from build123d import *

# Parameters (mm, degrees)
SKETCH1_W           = 152.4
SKETCH1_H           = 76.2
BOSS_EXTRUDE1_DEPTH = 6.35
SKETCH2_W           = 6.35
SKETCH2_H           = 38.1
BOSS_EXTRUDE2_DEPTH = 6.35
CUT_EXTRUDE1_DEPTH  = 7.35
CUT_EXTRUDE2_DEPTH  = 7.35
BOSS_EXTRUDE3_DEPTH = 6.35
CUT_EXTRUDE3_DEPTH  = 7.35
FILLET1_R           = 48.26
CUT_EXTRUDE4_DEPTH  = 7.35
EXTRUDE_THIN2_DEPTH = 6.35
FILLET2_R           = 3.175


with BuildPart() as part:
    # Sketch1 → Boss-Extrude1 (new body)
    with BuildSketch(Plane.XY):
        with Locations((-76.2, -38.1)):
            Rectangle(SKETCH1_W, SKETCH1_H)
    extrude(amount=BOSS_EXTRUDE1_DEPTH)

    # Sketch2 → Boss-Extrude2 (add)
    with BuildSketch(Plane.XY.offset(6.35)):
        with Locations((3.175, -38.1)):
            Rectangle(SKETCH2_W, SKETCH2_H)
    extrude(amount=-BOSS_EXTRUDE2_DEPTH)

    # Sketch3 → Cut-Extrude1 (cut, through all)
    with BuildSketch(Plane.XY.offset(6.35)):
        Polygon((-152.4, -59.878913996), (-70.683723912, -12.7), (-12.7, -12.7), (-12.7, 0), (-152.4, 0), align=None)
    extrude(amount=-CUT_EXTRUDE1_DEPTH, mode=Mode.SUBTRACT)

    # Sketch4 → Cut-Extrude2 (cut, through all)
    with BuildSketch(Plane.XY.offset(6.35)):
        Polygon((-152.4, -59.878913996), (-133.35, -76.2), (-152.4, -76.2), align=None)
    extrude(amount=-CUT_EXTRUDE2_DEPTH, mode=Mode.SUBTRACT)

    # Sketch5 → Boss-Extrude3 (add)
    with BuildSketch(Plane.XY.offset(6.35)):
        Polygon((-87.181507854, -22.225), (-90.356507854, -16.725738686), (-123.352075739, -35.775738686), (-120.177075739, -41.275), align=None)
    extrude(amount=-BOSS_EXTRUDE3_DEPTH)

    # Sketch6 → Cut-Extrude3 (cut, through all)
    with BuildSketch(Plane.XY.offset(6.35)):
        Polygon((-134.802363795, -49.718913996), (-119.513501663, -76.2), (-133.35, -76.2), (-152.4, -59.878913996), align=None)
    extrude(amount=-CUT_EXTRUDE3_DEPTH, mode=Mode.SUBTRACT)

    # Fillet1
    fillet1_edges = [part.edges().sort_by_distance(p)[0] for p in [
        (-119.513501663, -76.2, 3.175),
    ]]
    fillet(fillet1_edges, radius=FILLET1_R)

    # Sketch7 → Cut-Extrude4 (cut, through all)
    with BuildSketch(Plane.XY.offset(6.35)):
        with BuildLine():
            Line((-102.82855311, -45.923522628), (-91.830030482, -39.573522628))
            Line((-91.830030482, -39.573522628), (-67.280769168, -25.4))
            Line((-67.280769168, -25.4), (-12.7, -25.4))
            Line((-12.7, -25.4), (-12.7, -31.75))
            Line((-12.7, -31.75), (-12.7, -44.45))
            Line((-12.7, -44.45), (-12.7, -63.5))
            Line((-12.7, -63.5), (-91.650577671, -63.5))
            ThreePointArc((-91.650577671, -63.5), (-104.882957084, -60.946328713), (-116.214822021, -53.652088587))
            Line((-116.214822021, -53.652088587), (-102.82855311, -45.923522628))
        make_face()
    extrude(amount=-CUT_EXTRUDE4_DEPTH, mode=Mode.SUBTRACT)

    # Sketch8 → Extrude-Thin2 (add)
    with BuildSketch(Plane.XY.offset(6.35)):
        Polygon((-9.974003812, -59.594830217), (-72.043269168, -16.267499985), (-72.043269168, -63.5), (-62.518269168, -63.5), (-62.518269168, -34.532500015), (-15.425996188, -67.405169783), align=None)
    extrude(amount=-EXTRUDE_THIN2_DEPTH)

    # Fillet2
    fillet2_edges = [part.edges().sort_by_distance(p)[0] for p in [
        (-116.214822021, -53.652088587, 3.175),
        (-12.7, -25.4, 3.175),
        (-21.020410111, -63.5, 3.175),
        (-12.7, -57.691953868, 3.175),
        (-58.960359057, -25.4, 3.175),
        (-72.043269168, -63.5, 3.175),
        (-72.043269168, -28.149630657, 3.175),
        (-62.518269168, -34.532500015, 3.175),
        (-62.518269168, -63.5, 3.175),
    ]]
    fillet(fillet2_edges, radius=FILLET2_R)


solid = part.part
Read the model definition and answer for the solid it produces. Units are mm, in the model's axes. A direction names the side the tool comes from. Round coordinates to 2 decimals unless told otherwise and drop trailing zeros. Order: outer loops, then holes, each group sorted by start corner. A loop starts at its lowest first (then second) coordinate and runs counter-clockwise, first axis right, second up. Notation, with made-up numbers: (66, -28.5) - (124, -28.5) arc R31 cw to (124, 0.5) - close; hole circle Ø11 at (83, 83.25). An arc over 180 degrees is marked (long way). Use one line per item in the form item = value. Start each with the question number.
(1) The part is cut by section A-A (x = -20.5). Give the vertices of the cut face in (y, z), then the cut area to 3 significant figures.
(2) The part is cut by section D-D (y = -6). Give the vertices of the cut face in (x, z), then the cut area to 3 significant figures.
(3) Determine the mould class of faces 6 (the face through (-45, -63.5, 3)), 7 (the face through (0, -10, 3)), 8 (the face through (-50, -38, 6.35)), 9 (the face through (-127.592, -45.556, 3.219)) for opening direction X: +X half, -X half, draft (parallel to the pull), parting line (faces both ways), or undercut.
(4) Flat-ended cylindrical pins translate along their axes: pin 1 Ø1.9 at (y, z) = (-44, 2) entering from -X; pin 2 Ø3 at (y, z) = (-9, 2.5) entering from +X; pin 3 Ø1 at (x, z) = (-19.5, 4.5) entering from +Y. Find the tip coordinate at first contact, or state that the pin passes through.
(5) Find the intervals of material crossed by line 1 along Y through (x, z) = (-16, 5.5); line 2 along X through (y, z) = (-55.5, 2.5); line 3 along X through (y, z) = (-57, 3.25), in increasing order. Write a range as from..to.
(6) The part is cut by section C-C (x = -69). Give the vertices of the cut face in (y, z).
(7) For faces 1 (the face through (3, -57.15, 3)), 2 (the face through (-42, -12.7, 3)), 3 (the face through (3, -19.05, 3)), 4 (the face through (-79, -17.5, 3.2)), 5 (the face through (-72.043, -47, 3)), determine the directions among +Z, -Z, +X, -X, +Y, -Y from which every point of the face is accessible in a straight line to the end or side of a thin tool.
(8) The part is cut by section B-B (z = 4.5). Count the separate pieces of the cut face and the enclosed holes in it, then the cut area to 3 significant figures.
Checked values:
q1.outline = (-76.2, 0) - (-52.25, 0) - (-52.25, 6.35) - (-76.2, 6.35) - close; (-25.4, 0) - (-12.7, 0) - (-12.7, 6.35) - (-25.4, 6.35) - close
q1.area = 233 mm^2
q2.outline = (-12.7, 0) - (0, 0) - (0, 6.35) - (-12.7, 6.35) - close
q2.area = 80.6 mm^2
q3.face_6 = undercut
q3.face_7 = +X half
q3.face_8 = draft
q3.face_9 = -X half
q4.pin_1 = -126.54
q4.pin_2 = 0
q4.pin_3 = -12.7
q5.line_1 = -76.2..-54.78, -25.4..-12.7
q5.line_2 = -131.27..-113.56, -72.04..-62.52, -32.48..6.35
q5.line_3 = -130.18..-112.15, -72.04..-62.52, -30.33..6.35
q6.outline = (-76.2, 0) - (-12.7, 0) - (-12.7, 6.35) - (-76.2, 6.35) - close
q7.face_1 = +Z, -Z, +X, -Y
q7.face_2 = +Z, -Z, -X, +Y
q7.face_3 = +Z, -Z, +X, +Y
q7.face_4 = +Z, -Z, +Y
q7.face_5 = +Z, -Z
q8.separate_pieces = 1
q8.enclosed_holes = 3
q8.area = 5,490 mm^2
